Geometry check sheet. Reference: the model listing, model coordinates, mm. A direction names the side the tool comes from. Coordinates: 2 decimals unless noted, no trailing zeros. Order: outer loops, then holes, each group sorted by start corner. A loop starts at its lowest first (then second) coordinate and runs counter-clockwise, first axis right, second up. Notation, with made-up numbers: (2, 31) - (12, 31) arc R18 ccw to (12, 45) - close; hole circle Ø7 at (-2, 58.5). An arc over 180 degrees is marked (long way). Put each result on its own line as item: value.
from build123d import *

# Parameters (mm, degrees)
SKETCH1_W           = 20
SKETCH1_H           = 35
SKETCH1_R           = 3.3734375
BOSS_EXTRUDE1_DEPTH = 5
SKETCH2_W           = 20
SKETCH2_H           = 5
BOSS_EXTRUDE2_DEPTH = 20
SKETCH3_R           = 3.3734375
BOSS_EXTRUDE3_DEPTH = 20
SKETCH4_W           = 20
SKETCH4_H           = 35
CUT_EXTRUDE1_DEPTH  = 5
BOSS_EXTRUDE4_START = -3
SKETCH5_R           = 3.3734375
BOSS_EXTRUDE4_DEPTH = 3
SKETCH6_W           = 10
SKETCH6_H           = 7
SKETCH6_R           = 1.3
BOSS_EXTRUDE5_DEPTH = 5
FILLET1_R           = 3


with BuildPart() as part:
    # Sketch1 → Boss-Extrude1 (new body)
    with BuildSketch(Plane(origin=(0, 0, 0), x_dir=(1, 0, 0), z_dir=(0, 1, 0))):
        with Locations((10, 17.5)):
            Rectangle(SKETCH1_W, SKETCH1_H)
        with Locations(Location((10, 26.15, 0), (0, 0, 270))):
            Circle(SKETCH1_R, mode=Mode.SUBTRACT)
    extrude(amount=BOSS_EXTRUDE1_DEPTH)

    # Sketch2 → Boss-Extrude2 (add)
    with BuildSketch(Plane(origin=(0, 5, 0), x_dir=(1, 0, 0), z_dir=(0, 1, 0))):
        with Locations((10, 2.5)):
            Rectangle(SKETCH2_W, SKETCH2_H)
    extrude(amount=BOSS_EXTRUDE2_DEPTH)

    # Sketch3 → Boss-Extrude3 (add)
    with BuildSketch(Plane(origin=(0, 5, 0), x_dir=(1, 0, 0), z_dir=(0, 1, 0))):
        with BuildLine():
            Line((5, 5), (15, 5))
            ThreePointArc((15, 5), (12.311517531, 13.916687605), (15, 22.83337521))
            ThreePointArc((15, 22.83337521), (10, 32.15), (5, 22.83337521))
            ThreePointArc((5, 22.83337521), (7.688482469, 13.916687605), (5, 5))
        make_face()
        with Locations(Location((10, 26.15, 0), (0, 0, 270))):
            Circle(SKETCH3_R, mode=Mode.SUBTRACT)
    extrude(amount=BOSS_EXTRUDE3_DEPTH)

    # Sketch4 → Cut-Extrude1 (cut)
    with BuildSketch(Plane.XZ):
        with Locations((10, -17.5)):
            Rectangle(SKETCH4_W, SKETCH4_H)
    extrude(amount=-CUT_EXTRUDE1_DEPTH, mode=Mode.SUBTRACT)

    # Sketch5 → Boss-Extrude4 (add)
    with BuildSketch(Plane(origin=(0, 25, 0), x_dir=(1, 0, 0), z_dir=(0, 1, 0)).offset(BOSS_EXTRUDE4_START)):
        with Locations(Location((10, 26.15, 0), (0, 0, 90))):
            Circle(SKETCH5_R)
    extrude(amount=BOSS_EXTRUDE4_DEPTH)

    # Sketch6 → Boss-Extrude5 (add)
    # profile 1 of 2: a face of its own
    with BuildSketch(Plane.XY):
        with Locations((25, 8.5)):
            Rectangle(SKETCH6_W, SKETCH6_H)
        with Locations((27, 8.5)):
            Circle(SKETCH6_R, mode=Mode.SUBTRACT)
    # profile 2 of 2: a face of its own
    with BuildSketch(Plane.XY):
        with Locations((-5, 21.5)):
            Rectangle(SKETCH6_W, SKETCH6_H)
        with Locations((-7, 21.5)):
            Circle(SKETCH6_R, mode=Mode.SUBTRACT)
    extrude(amount=-BOSS_EXTRUDE5_DEPTH)

    # Fillet1
    fillet1_edges = [part.edges().sort_by_distance(p)[0] for p in [
        (20, 25, -2.5),
        (5, 15, -5),
        (15, 15, -5),
        (0, 5, -2.5),
        (30, 5, -2.5),
        (30, 12, -2.5),
        (20, 12, -2.5),
        (-10, 25, -2.5),
        (-10, 18, -2.5),
        (0, 18, -2.5),
    ]]
    fillet(fillet1_edges, radius=FILLET1_R)


solid = part.part
Q1. Section check A-A on y = 21.5. Record the boundary of the cut face in (x, z).
Answer block:
outline: (-10, -5) - (-8.3, -5) - (-8.3, 0) - (-10, 0) - close; (-5.7, -5) - (3.28, -5) arc R3 cw to (5.96, -6.65) arc R16.13 cw to (5, -22.83) arc R6 ccw (long way) to (15, -22.83) arc R16.13 cw to (14.04, -6.65) arc R3 cw to (16.72, -5) - (20, -5) - (20, 0) - (-5.7, 0) - close; hole circle Ø6.75 at (10, -26.15)
Q2. Section check D-D on x = 14.5. Record the boundary of the cut face in (y, z).
Answer block:
outline: (5, -30.12) - (25, -30.12) - (25, -22.03) - (5, -22.03) - close; (5, -5.98) - (25, -5.98) - (25, 0) - (5, 0) - close
Q3. Section check B-B on z = -3. Record the boundary of the cut face in (x, y), then the cut area to 3 significant figures.
Answer block:
outline: (-10, 21) arc R3 ccw to (-7, 18) - (-3, 18) arc R3 cw to (0, 15) - (0, 8) arc R3 ccw to (3, 5) - (27, 5) arc R3 ccw to (30, 8) - (30, 9) arc R3 ccw to (27, 12) - (23, 12) arc R3 cw to (20, 15) - (20, 22) arc R3 ccw to (17, 25) - (-7, 25) arc R3 ccw to (-10, 22) - close; hole circle Ø2.6 at (-7, 21.5); hole circle Ø2.6 at (27, 8.5)
area: 522 mm^2
Q4. Section check C-C on z = -26.15. Record the boundary of the cut face in (x, y).
Answer block:
outline: (4, 5) - (6.63, 5) - (6.63, 22) - (13.37, 22) - (13.37, 5) - (16, 5) - (16, 25) - (4, 25) - close
Q5. Draft check along X on faces 4 (the cylindrical face through (10.181, 14.86, -32.147)), 5 (the flat face through (10, 25, -16)), 6 (the cylindrical face through (13.345, 13.381, -26.589)). Enter one of: pulls with the +X half, pulls with the -X half, needs draft (parallel to the pull), parting line crosses it, or undercut.
Answer block:
face 4: parting line crosses it
face 5: needs draft
face 6: undercut
Q6. Access from +Z, -Z, +X, -X, +Y, -Y to the whole of each face (thin tool, end or side, straight path). Record for faces 1 (the cylindrical face through (4.872, 15.14, -5.457)), 2 (the flat face through (20, 18, -2)), 3 (the cylindrical face through (15.17, 15.14, -5.43)).
Answer block:
face 1: -X, +Y, -Y
face 2: +Z, -Z, +X, +Y
face 3: +X, +Y, -Y
Q7. Depth check by flat-ended pin: pin 1 Ø8 at (y, z) = (7.5, -3.5) entering from +X; pin 2 Ø1.5 at (y, z) = (19.5, -10.5) entering from -X; pin 3 Ø4 at (y, z) = (19, -17) entering from -X; pin 4 Ø2 at (x, z) = (25.5, -3.5) entering from +Y. Enter the tip coordinate at first touch or a pass-through.
Answer block:
pin 1: stops at x = 30
pin 2: stops at x = 7.14
pin 3: stops at x = 6.87
pin 4: stops at y = 12
Q8. Thickness scan on L1, parallel to Z at x = 10, y = 11.5; L2, parallel to X at y = 9.5, z = -26.15; L3, parallel to X at y = 15, z = -28. Record the ranges inside material, lowest first. Write a range as [from, to].
Answer block:
L1: z = [-32.15, -29.52], [-22.78, 0]
L2: x = [4, 6.63], [13.37, 16]
L3: x = [4.29, 7.18], [12.82, 15.71]
